Can you work these out from the drawing? Everything is in mm from the part's minimum corner. A direction names the side the tool comes from. Give positions to 0.01 mm unless a question says otherwise; leave off trailing zeros. Order: outer loops, then holes, each group sorted by start corner. A loop starts at its lowest first (then second) coordinate and runs counter-clockwise, first axis right, second up. Notation, with made-up numbers: (88.5, -10) - (97.5, -10) arc R11 cw to (97.5, -6) - close; hole circle Ø5 at (44, 55.5). An arc over 180 degrees is marked (long way). One line per question, with ' | ' between items.
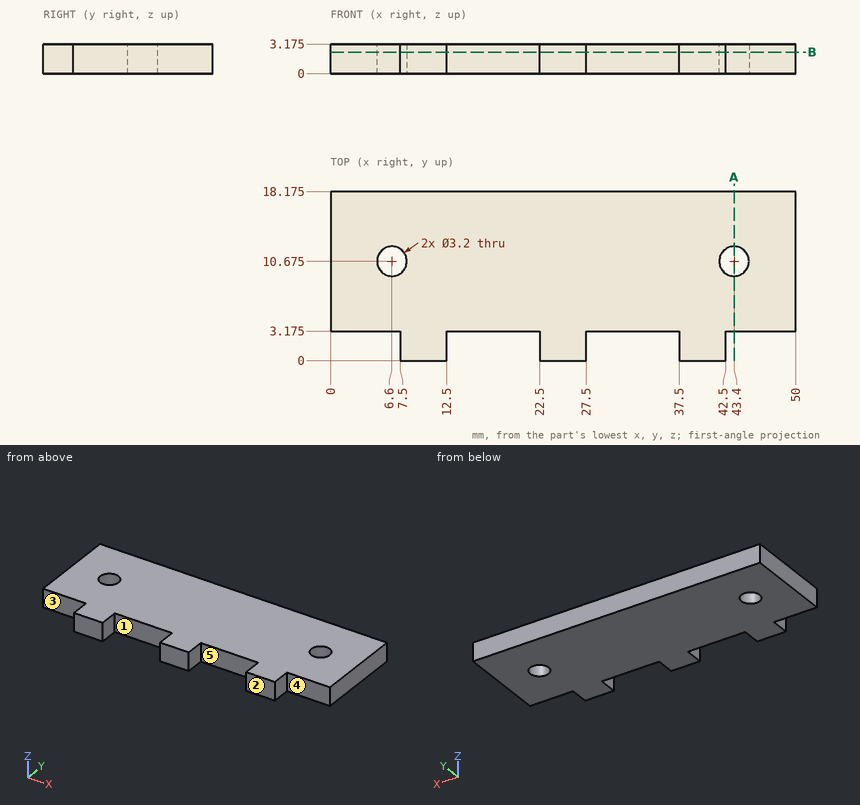
(1) Will these pins go through, and if not, where does the flat tip stop? pin 1 (1.6 mm diameter, centred on y = 1.5, z = 1, fed in from -X); pin 2 (1 mm diameter, centred on y = 2, z = 2, fed in from +X); pin 3 (1 mm diameter, centred on x = 46.5, z = 1.5, fed in from -Y) (3 decimals).
Answer below:
pin 1: x = 7.5 | pin 2: x = 42.5 | pin 3: y = 3.175
(2) Imagine slicing it at A-A (x = 43.4). List the corners of the cut face in (y, z) for me (3 decimals), and give its area (3 significant figures).
Answer below:
outline: (3.175, 0) - (9.075, 0) - (9.075, 3.175) - (3.175, 3.175) - close; (12.275, 0) - (18.175, 0) - (18.175, 3.175) - (12.275, 3.175) - close | area: 37.5 mm^2
(3) On a 3-axis mill with a long thin cutter (end or side, diameter ignored), from which of +Z, -Z, +X, -X, +Y, -Y can I reach the whole of each face in a straight line? I mean the marked faces 1, 2 and 3. Say none if no direction works.
Answer below:
face 1: +Z, -Z, -Y | face 2: +Z, -Z, +X, -X, -Y | face 3: +Z, -Z, -X, -Y
(4) If we mould it in two halves opening along X, with no side actions, what happens to the marked faces 4 and 5? For each: released by +X, released by -X, zero draft, split by the parting line, or undercut.
Answer below:
face 4: zero draft | face 5: undercut
(5) Imagine slicing it at B-B (z = 2.3). List the corners of the cut face in (x, y) for me (3 decimals).
Answer below:
outline: (0, 3.175) - (7.5, 3.175) - (7.5, 0) - (12.5, 0) - (12.5, 3.175) - (22.5, 3.175) - (22.5, 0) - (27.5, 0) - (27.5, 3.175) - (37.5, 3.175) - (37.5, 0) - (42.5, 0) - (42.5, 3.175) - (50, 3.175) - (50, 18.175) - (0, 18.175) - close; hole circle Ø3.2 at (6.6, 10.675); hole circle Ø3.2 at (43.4, 10.675)
(6) If I drill on line 1 (X direction, y = 10.25, z = 0.5); line 2 (Y direction, x = 43.4, z = 0.95) (3 decimals); line 3 (Y direction, x = 29, z = 2.9) (3 decimals), over which ranges is the centre line in solid material (lowest first)?
Answer below:
line 1: 0 to 5.06, 8.14 to 41.86, 44.94 to 50 | line 2: 3.175 to 9.075, 12.275 to 18.175 | line 3: 3.175 to 18.175
